Autodesk Inventor part; units mm, degrees
ref_plane "YZ Plane" through (0, 0, 0) normal (1, 0, 0) x (0, 1, 0)
ref_plane "XZ Plane" through (0, 0, 0) normal (0, 1, 0) x (-1, 0, 0)
ref_plane "XY Plane" through (0, 0, 0) normal (0, 0, 1) x (1, 0, 0)
sketch "Sketch1" plane through (0, 0, 0) normal (0, 1, 0) x (-1, 0, 0)
  line L0 (40, -150) -> (-40, -150)
  line L1 (-40, -150) -> (-40, 150)
  line L2 (-40, 150) -> (40, 150)
  line L3 (40, 150) -> (40, -150)
  line L4 (0, -150) -> (0, 150)
  line L5 (40, 0) -> (-40, 0)
  point P0 (0, 0)
  dimension "d0" = 300
  dimension "d1" = 80
extrude "Extrusion1" add sketch "Sketch1" along normal blind 0.1
sketch "Sketch2" plane through (0, 0.1, 0) normal (0, 1, 0) x (1, 0, 0)
  line L0 (-40, -150) -> (40, -150)
  line L1 (40, -150) -> (40, 150)
  line L2 (40, 150) -> (-40, 150)
  line L3 (-40, 150) -> (-40, -150)
  line L4 (-27.5, 175) -> (-27.5, -125)
  line L5 (-27.5, -125) -> (27.5, -125)
  line L6 (27.5, -125) -> (27.5, 125)
  line L7 (27.5, 125) -> (-14.8, 125)
  line L8 (-14.8, 125) -> (-14.8, 175)
  line L9 (-14.8, 175) -> (-27.5, 175)
  line L10 (-14.8, 112.3) -> (-14.8, 6.35)
  line L11 (-14.8, 6.35) -> (14.8, 6.35)
  line L12 (14.8, 6.35) -> (14.8, 112.3)
  line L13 (14.8, 112.3) -> (-14.8, 112.3)
  line L14 (-14.8, -6.35) -> (14.8, -6.35)
  line L15 (14.8, -6.35) -> (14.8, -112.3)
  line L16 (14.8, -112.3) -> (-14.8, -112.3)
  line L17 (-14.8, -112.3) -> (-14.8, -6.35)
  line L18 (-40, 0) -> (40, 0)
  point P0 (0, 0)
  dimension "d4" = 12.7
  dimension "d5" = 12.7
  dimension "d6" = 12.7
  dimension "d7" = 12.7
  dimension "d8" = 12.7
  dimension "d9" = 25
  dimension "d10" = 25
  dimension "d11" = 12.5
  dimension "d12" = 12.5
  dimension "d13" = 250
  dimension "d14" = 50
extrude "Extrusion2" add sketch "Sketch2" along normal blind 0.1 contours L18 L6 L5 L4 | L4 L2 L8 L7 L6 L18 | L4 L9 L8 L2
sketch "Sketch3" plane through (0, 0, 0) normal (0, -1, 0) x (1, 0, 0)
  line L0 (40, -150) -> (-40, -150)
  line L1 (27.5, 125) -> (27.5, -175)
  line L2 (27.5, -175) -> (14.8, -175)
  line L3 (14.8, -175) -> (14.8, -125)
  line L4 (14.8, -125) -> (-27.5, -125)
  line L5 (-27.5, -125) -> (-27.5, 125)
  line L6 (-27.5, 125) -> (27.5, 125)
  line L7 (-14.8, 112.3) -> (14.8, 112.3)
  line L8 (14.8, 112.3) -> (14.8, 6.35)
  line L9 (14.8, 6.35) -> (-14.8, 6.35)
  line L10 (-14.8, 6.35) -> (-14.8, 112.3)
  line L11 (-14.8, -6.35) -> (14.8, -6.35)
  line L12 (14.8, -6.35) -> (14.8, -112.3)
  line L13 (14.8, -112.3) -> (-14.8, -112.3)
  line L14 (-14.8, -112.3) -> (-14.8, -6.35)
  line L15 (27.5, 125) -> (-27.5, 125)
  line L16 (-14.8, 112.3) -> (14.8, 112.3)
  line L17 (-27.5, 125) -> (-27.5, -150)
  line L18 (27.5, -125) -> (27.5, 125)
  line L19 (-14.8, -125) -> (27.5, -125)
  line L20 (14.8, -6.35) -> (14.8, -112.3)
  line L21 (-14.8, -112.3) -> (-14.8, -6.35)
  line L22 (-14.8, -6.35) -> (14.8, -6.35)
  line L23 (14.8, 6.35) -> (-14.8, 6.35)
  line L24 (14.8, -112.3) -> (-14.8, -112.3)
  line L25 (-14.8, -175) -> (-27.5, -175)
  point P0 (0, 0)
extrude "Extrusion3" add sketch "Sketch3" along normal blind 0.1 contours L1 L2 L3 L0 | L0 L3 L19 L1 | L19 L4 L5 L6 L1
properties part number "Captor"
Could you check a few things on this model? Use its own coordinates, in mm. Round coordinates to 2 decimals unless told otherwise and drop trailing zeros. Loops run counter-clockwise (first coordinate to the right, second up) from the corner with the lowest first, then second, coordinate; pieces in that order, holes last. Notation, with made-up numbers: M -34,19.5 L 6,19.5 A9 ccw 6,30.5 Z; hole C 32.25,7 d9. An arc over 180 degrees is marked long. Write item = value, one per line.
1. I need wall thicknesses on probe 1 along X at (y, z) = (-0.05, -17.5); probe 2 along Z at (x, y) = (11, 0.05). Which ranges of each line are inside material? Lowest first, please.
Results below:
probe_1 = -27.5 to -14.8, 14.8 to 27.5
probe_2 = -150 to 150
2. I want a section at B-B, the plane x = 12. Write out the boundary of the cut face in (y, z).
Results below:
outline = M -0.1,-125 L 0,-125 L 0,-150 L 0.1,-150 L 0.1,-125 L 0.2,-125 L 0.2,-112.3 L 0.1,-112.3 L 0.1,-6.35 L 0.2,-6.35 L 0.2,6.35 L 0.1,6.35 L 0.1,112.3 L 0.2,112.3 L 0.2,125 L 0.1,125 L 0.1,150 L 0,150 L 0,125 L -0.1,125 L -0.1,112.3 L 0,112.3 L 0,6.35 L -0.1,6.35 L -0.1,-6.35 L 0,-6.35 L 0,-112.3 L -0.1,-112.3 Z
3. I want a section at D-D, the plane z = -138. Write out the boundary of the cut face in (x, y).
Results below:
outline = M -40,0 L 14.8,0 L 14.8,-0.1 L 27.5,-0.1 L 27.5,0 L 40,0 L 40,0.1 L -14.8,0.1 L -14.8,0.2 L -27.5,0.2 L -27.5,0.1 L -40,0.1 Z
4. I want a section at A-A, the plane y = 0.15. Write out the boundary of the cut face in (x, z).
Results below:
outline = M -27.5,-175 L -14.8,-175 L -14.8,-125 L 27.5,-125 L 27.5,125 L -27.5,125 Z; hole M -14.8,-112.3 L 14.8,-112.3 L 14.8,-6.35 L -14.8,-6.35 Z; hole M -14.8,6.35 L 14.8,6.35 L 14.8,112.3 L -14.8,112.3 Z
5. I want a section at C-C, the plane z = 80.5. Write out the boundary of the cut face in (x, y), and give its area (3 significant figures).
Results below:
outline = M -40,0 L -27.5,0 L -27.5,-0.1 L -14.8,-0.1 L -14.8,0 L 14.8,0 L 14.8,-0.1 L 27.5,-0.1 L 27.5,0 L 40,0 L 40,0.1 L 27.5,0.1 L 27.5,0.2 L 14.8,0.2 L 14.8,0.1 L -14.8,0.1 L -14.8,0.2 L -27.5,0.2 L -27.5,0.1 L -40,0.1 Z
area = 13.1 mm²
6. Will these pins go through, and if not, where does the flat tip stop? P1, Ø6.5, axis at x = 20.5, z = -167, coming from the +Y side; P2, Ø3, axis at x = 6, z = -12, coming from the +Y side; P3, Ø5, axis at x = 11.5, z = 87, coming from the -Y side.
Results below:
P1 = 0
P2 = 0.1
P3 = 0
